from build123d import *

# Parameters (mm, degrees)
F3_DEPTH = 25.4
F4_DEPTH = 38.1
F5_DEPTH = 25.4


with BuildPart() as f3:
    # F0 (on Front) → F3 (new body)
    with BuildSketch(Plane.XZ):
        Polygon((0, 25.4), (0, 0), (38.171803, 0), (38.171803, 6.314098), (12.7, 6.314098), (12.7, 19.05), (12.7, 25.4), align=None)
    extrude(amount=-F3_DEPTH)

    # F1 (on Right) → F4 (join)
    with BuildSketch(Plane.YZ):
        Polygon((0, 6.35), (0, 0), (25.4, 0), (25.4, 19.05), (19.05, 19.05), (19.05, 6.35), align=None)
    extrude(amount=F4_DEPTH)

    # F2 (on Top) → F5 (join)
    with BuildSketch(Plane.XY):
        Polygon((0, 25.4), (0, 0), (12.673074, 0), (12.673074, 19.05), (38.073074, 19.05), (38.1, 25.4), align=None)
    extrude(amount=F5_DEPTH)


solid = f3.part
The model under review builds one solid part; all positions refer to its coordinate system, in mm. A direction names the side the tool comes from. Round coordinates to 2 decimals unless told otherwise and drop trailing zeros. Loops run counter-clockwise (first coordinate to the right, second up) from the corner with the lowest first, then second, coordinate; pieces in that order, holes last. Notation, with made-up numbers: M 10,62 L 36,62 A21 ccw 36,81 Z; hole C 38,88.5 d6. An arc over 180 degrees is marked long. Answer as CSV lines item,"result".
1. We need section C-C (x = 16.5). Give the boundary of the cut face in (y, z).
Outcome:
outline,"M 0,0 L 25.4,0 L 25.4,25.4 L 19.05,25.4 L 19.05,6.35 L 0,6.35 Z"
2. To check wall thickness, follow L1, parallel to Y at x = 15.5, z = 9; L2, parallel to X at y = 21.75, z = 19.75; L3, parallel to X at y = 4.5, z = 15.75. State the ranges of each line that lie inside material, in increasing order. Write a range as [from, to].
Outcome:
L1,"y = [19.05, 25.4]"
L2,"x = [0, 38.08]"
L3,"x = [0, 12.7]"
3. We need section A-A (z = 15.75). Give the boundary of the cut face in (x, y).
Outcome:
outline,"M 0,0 L 12.7,0 L 12.7,19.05 L 38.1,19.05 L 38.1,25.4 L 0,25.4 Z"
4. For faces 1 (the face through (25, 19.05, 16)), 2 (the face through (38.172, 13, 3)), 3 (the face through (38.1, 22, 13)), list the 3-axis set-ups (+Z, -Z, +X, -X, +Y, -Y) from which the entire face can be reached by the end or side of a thin tool; tool diameter is ignored.
Outcome:
face 1,"+Z, +X, -Y"
face 2,"+Z, -Z, +X, +Y, -Y"
face 3,"+Z, +X, +Y, -Y"
5. Insertion check: pin 1 Ø3 at (x, y) = (28, 10) entering from +Z; pin 2 Ø9.5 at (y, z) = (9.5, 12.5) entering from +X. Each pin has a flat end and moves straight along its axis. Give the tip position at first contact, or say it passes through.
Outcome:
pin 1,"stops at z = 6.35"
pin 2,"stops at x = 12.7"
